Answer from the drawing. Dimensions are ordinates in mm from the lowest x, y and z of the part. Round coordinates to 2 decimals unless told otherwise and drop trailing zeros. Write each loop counter-clockwise with the first axis right and the second up, starting at its lowest first coordinate (ties: lowest second). Pieces come first, ordered by that corner, then holes. Notation, with made-up numbers: (35.25, 55.25) -> (55.25, 55.25) arc R11 cw to (55.25, 63.25) -> close; hole circle Ø5 at (49.25, 86). An arc over 180 degrees is marked (long way). Return JSON: item names as keys, results as strings. Group by question number.
(1) A cutting plane is placed at C-C on x = 83. Give the vertices of the cut face in (y, z) (3 decimals).
(2) A cutting plane is placed at B-B on x = 44.45. Give the vertices of the cut face in (y, z) (3 decimals), then the cut area to 3 significant figures.
(3) Given pin 1 (13.5 mm diameter, centred on x = 44.45, z = 25.4, fed in from +Y) (3 decimals); pin 2 (1 mm diameter, centred on y = 1, z = 19.5, fed in from -X), each flat-ended and moving along its own axis, determine where each tip first touches the part or whether it passes through.
(4) A cutting plane is placed at A-A on y = 0.65. Give the vertices of the cut face in (x, z), then the cut area to 3 significant figures.
(5) Straight lines are drawn through the part: line 1 (Z direction, x = 25, y = 1.85); line 2 (X direction, y = 1.2, z = 31.5); line 3 (X direction, y = 1.8, z = 15). For each, find the intervals that lie inside material, in ascending order.
(6) A cutting plane is placed at D-D on z = 47. Give the vertices of the cut face in (x, y) (3 decimals).
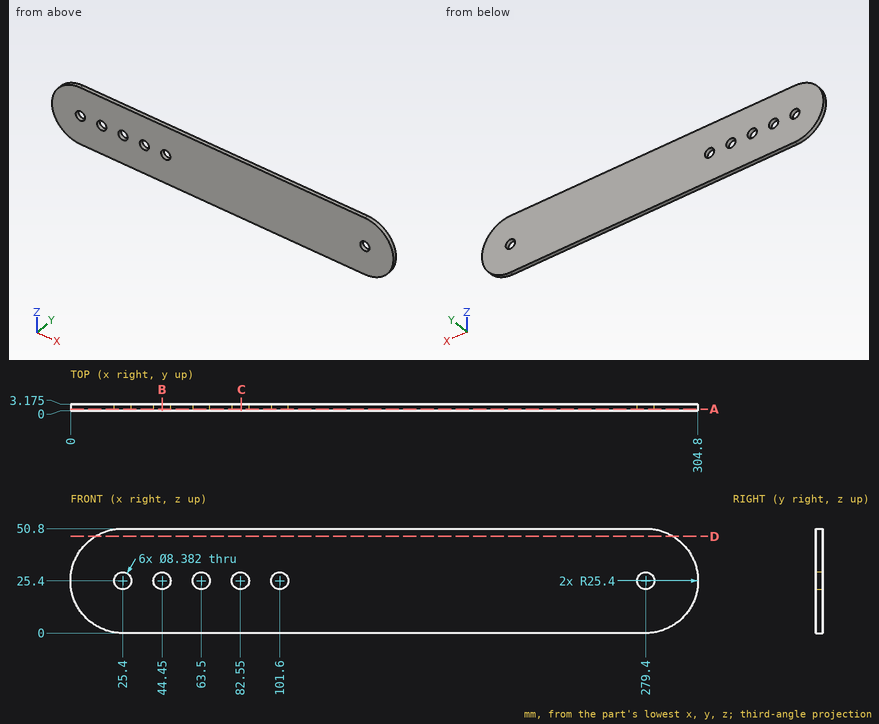
Checks:
{
 "1": {"outline": "(0, 0) -> (3.175, 0) -> (3.175, 21.233) -> (0, 21.233) -> close; (0, 29.567) -> (3.175, 29.567) -> (3.175, 50.8) -> (0, 50.8) -> close"},
 "2": {"outline": "(0, 0) -> (3.175, 0) -> (3.175, 21.209) -> (0, 21.209) -> close; (0, 29.591) -> (3.175, 29.591) -> (3.175, 50.8) -> (0, 50.8) -> close", "area": "135 mm^2"},
 "3": {"pin 1": "stops at y = 3.175", "pin 2": "stops at x = 0.58"},
 "4": {"outline": "(25.4, 0) -> (279.4, 0) arc R25.4 ccw to (279.4, 50.8) -> (25.4, 50.8) arc R25.4 ccw to start; hole circle Ø8.38 at (25.4, 25.4); hole circle Ø8.38 at (44.45, 25.4); hole circle Ø8.38 at (63.5, 25.4); hole circle Ø8.38 at (82.55, 25.4); hole circle Ø8.38 at (101.6, 25.4); hole circle Ø8.38 at (279.4, 25.4)", "area": "14,600 mm^2"},
 "5": {"line 1": "z = 0 to 21.23, 29.57 to 50.8", "line 2": "x = 0.74 to 304.06", "line 3": "x = 2.23 to 302.57"},
 "6": {"outline": "(12.036, 0) -> (292.764, 0) -> (292.764, 3.175) -> (12.036, 3.175) -> close"}
}
